Could you check a few things on this model? Use its own coordinates, in mm. Face numbers are marked on the shaded views. A direction names the side the tool comes from. Round coordinates to 2 decimals unless told otherwise and drop trailing zeros. Write each loop counter-clockwise with the first axis right and the second up, starting at its lowest first coordinate (ties: lowest second). Pieces come first, ordered by that corner, then holes.
```python
from build123d import *

# Parameters (mm, degrees)
F1_DEPTH = 3.5
F2_DEPTH = 8
F3_DEPTH = 6


with BuildPart() as f1:
    # F0 (on Top) → F1 (new body)
    with BuildSketch(Plane.XY):
        with BuildLine():
            Line((1.05, -1.4), (1.75, -1.75))
            Line((1.75, -1.75), (1.75, 0))
            ThreePointArc((1.75, 0), (1.5652475842, -0.7826237921), (1.05, -1.4))
        make_face()
        Polygon((0, 1.75), (1.75, 1.75), (1.75, 3.75), (-1.75, 3.75), (-1.75, 1.75), align=None)
        Polygon((-1.75, -3.75), (1.75, -3.75), (1.75, -1.75), (0, -1.75), (-1.75, -1.75), align=None)
        with BuildLine():
            Line((0, -1.75), (1.75, -1.75))
            Line((1.75, -1.75), (1.05, -1.4))
            ThreePointArc((1.05, -1.4), (0.5533985905, -1.6601957716), (0, -1.75))
        make_face()
        with BuildLine():
            ThreePointArc((-1.75, 0), (-1.2374368671, -1.2374368671), (0, -1.75))
            ThreePointArc((0, -1.75), (0.5533985905, -1.6601957716), (1.05, -1.4))
            Line((1.05, -1.4), (-1.75, 0))
        make_face()
        with BuildLine():
            ThreePointArc((0, 1.75), (-1.2374368671, 1.2374368671), (-1.75, 0))
            Line((-1.75, 0), (1.05, 1.4))
            ThreePointArc((1.05, 1.4), (0.5533985905, 1.6601957716), (0, 1.75))
        make_face()
        with BuildLine():
            Line((1.05, 1.4), (1.75, 1.75))
            Line((1.75, 1.75), (0, 1.75))
            ThreePointArc((0, 1.75), (0.5533985905, 1.6601957716), (1.05, 1.4))
        make_face()
        with BuildLine():
            Line((-1.75, 0), (-1.75, -1.75))
            Line((-1.75, -1.75), (0, -1.75))
            ThreePointArc((0, -1.75), (-1.2374368671, -1.2374368671), (-1.75, 0))
        make_face()
        with BuildLine():
            ThreePointArc((1.05, -1.4), (1.5652475842, -0.7826237921), (1.75, 0))
            ThreePointArc((1.75, 0), (1.5652475842, 0.7826237921), (1.05, 1.4))
            Line((1.05, 1.4), (-1.75, 0))
            Line((-1.75, 0), (1.05, -1.4))
        make_face()
        with BuildLine():
            Line((-1.75, 1.75), (-1.75, 0))
            ThreePointArc((-1.75, 0), (-1.2374368671, 1.2374368671), (0, 1.75))
            Line((0, 1.75), (-1.75, 1.75))
        make_face()
        with BuildLine():
            ThreePointArc((1.05, 1.4), (1.5652475842, 0.7826237921), (1.75, 0))
            Line((1.75, 0), (1.75, 1.75))
            Line((1.75, 1.75), (1.05, 1.4))
        make_face()
    extrude(amount=F1_DEPTH)

    # F0 (on Top) → F2 (join)
    with BuildSketch(Plane.XY):
        with BuildLine():
            ThreePointArc((1.05, -1.4), (1.5652475842, -0.7826237921), (1.75, 0))
            ThreePointArc((1.75, 0), (1.5652475842, 0.7826237921), (1.05, 1.4))
            Line((1.05, 1.4), (-1.75, 0))
            Line((-1.75, 0), (1.05, -1.4))
        make_face()
        with BuildLine():
            ThreePointArc((-1.75, 0), (-1.2374368671, -1.2374368671), (0, -1.75))
            ThreePointArc((0, -1.75), (0.5533985905, -1.6601957716), (1.05, -1.4))
            Line((1.05, -1.4), (-1.75, 0))
        make_face()
        with BuildLine():
            ThreePointArc((0, 1.75), (-1.2374368671, 1.2374368671), (-1.75, 0))
            Line((-1.75, 0), (1.05, 1.4))
            ThreePointArc((1.05, 1.4), (0.5533985905, 1.6601957716), (0, 1.75))
        make_face()
    extrude(amount=F2_DEPTH)

    # F0 (on Top) → F3 (join)
    with BuildSketch(Plane.XY):
        with BuildLine():
            Line((0, -1.75), (1.75, -1.75))
            Line((1.75, -1.75), (1.05, -1.4))
            ThreePointArc((1.05, -1.4), (0.5533985905, -1.6601957716), (0, -1.75))
        make_face()
        with BuildLine():
            ThreePointArc((-1.75, 0), (-1.2374368671, -1.2374368671), (0, -1.75))
            ThreePointArc((0, -1.75), (0.5533985905, -1.6601957716), (1.05, -1.4))
            Line((1.05, -1.4), (-1.75, 0))
        make_face()
        with BuildLine():
            ThreePointArc((0, 1.75), (-1.2374368671, 1.2374368671), (-1.75, 0))
            Line((-1.75, 0), (1.05, 1.4))
            ThreePointArc((1.05, 1.4), (0.5533985905, 1.6601957716), (0, 1.75))
        make_face()
        with BuildLine():
            Line((1.05, 1.4), (1.75, 1.75))
            Line((1.75, 1.75), (0, 1.75))
            ThreePointArc((0, 1.75), (0.5533985905, 1.6601957716), (1.05, 1.4))
        make_face()
        with BuildLine():
            Line((1.05, -1.4), (1.75, -1.75))
            Line((1.75, -1.75), (1.75, 0))
            ThreePointArc((1.75, 0), (1.5652475842, -0.7826237921), (1.05, -1.4))
        make_face()
        with BuildLine():
            ThreePointArc((1.05, 1.4), (1.5652475842, 0.7826237921), (1.75, 0))
            Line((1.75, 0), (1.75, 1.75))
            Line((1.75, 1.75), (1.05, 1.4))
        make_face()
        with BuildLine():
            Line((-1.75, 0), (-1.75, -1.75))
            Line((-1.75, -1.75), (0, -1.75))
            ThreePointArc((0, -1.75), (-1.2374368671, -1.2374368671), (-1.75, 0))
        make_face()
        with BuildLine():
            Line((-1.75, 1.75), (-1.75, 0))
            ThreePointArc((-1.75, 0), (-1.2374368671, 1.2374368671), (0, 1.75))
            Line((0, 1.75), (-1.75, 1.75))
        make_face()
    extrude(amount=F3_DEPTH)


solid = f1.part
```
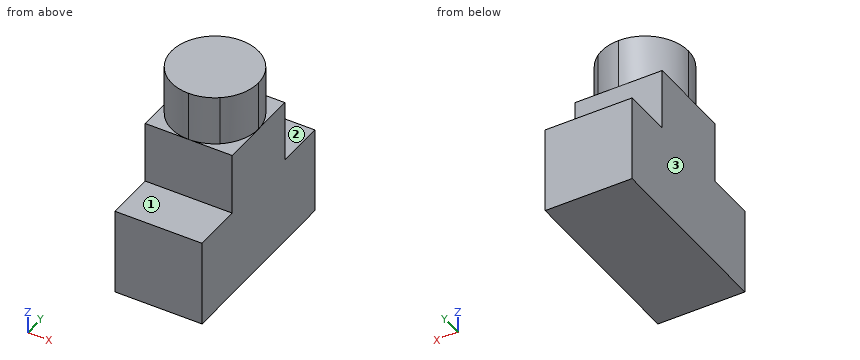
Q1. If I drill on L1, parallel to Y at x = 0.2, z = 5; L2, parallel to Z at x = -1.6, y = 2; L3, parallel to Z at x = -0.95, y = -1.5, over which ranges is the centre line in solid material (lowest first)?
Q2. On a 3-axis mill with a long thin cutter (end or side, diameter ignored), from which of +Z, -Z, +X, -X, +Y, -Y can I reach the whole of each face in a straight line? I mean the marked faces 1, 2 and 3. Say none if no direction works.
Q3. Imagine slicing it at C-C, the plane y = 0.75. Write out the boundary of the cut face in (x, z), then the cut area to 3 significant figures.
Q4. Imagine slicing it at A-A, the plane x = 1.4. Write out the boundary of the cut face in (y, z).
Q5. Imagine slicing it at D-D, the plane x = 0.45. Write out the boundary of the cut face in (y, z), then the cut area to 3 significant figures.
Q6. I'm going to push a flat-ended pin straight in: pin 1 Ø1 at (x, y) = (1, 3) entering from +Z. Where does the tip first touch, or does it pass through?
Q7. Imagine slicing it at B-B, the plane z = 7. Write out the boundary of the cut face in (x, y).
Results found:
1. L1: y = -1.75 to 1.75
1. L2: z = 0 to 3.5
1. L3: z = 0 to 6
2. face 1: +Z, +X, -X, -Y
2. face 2: +Z, +X, -X, +Y
2. face 3: +Z, -Z, -X, +Y, -Y
3. outline: (-1.75, 0) - (1.75, 0) - (1.75, 6) - (1.58, 6) - (1.58, 8) - (-1.58, 8) - (-1.58, 6) - (-1.75, 6) - close
3. area: 27.3 mm2
4. outline: (-3.75, 0) - (3.75, 0) - (3.75, 3.5) - (1.75, 3.5) - (1.75, 6) - (1.05, 6) - (1.05, 8) - (-1.05, 8) - (-1.05, 6) - (-1.75, 6) - (-1.75, 3.5) - (-3.75, 3.5) - close
5. outline: (-3.75, 0) - (3.75, 0) - (3.75, 3.5) - (1.75, 3.5) - (1.75, 6) - (1.69, 6) - (1.69, 8) - (-1.69, 8) - (-1.69, 6) - (-1.75, 6) - (-1.75, 3.5) - (-3.75, 3.5) - close
5. area: 41.8 mm2
6. pin 1: stops at z = 3.5
7. outline: circle Ø3.5 at (0, 0)
